Design review of the part built by this model. Coordinates are the model's own, in mm. Round coordinates to 2 decimals unless told otherwise and drop trailing zeros. Return JSON: item names as keys, results as strings. Group by question number.
(1) Clearance check with a flat-ended pin moving along its axis: pin 1 (6 mm diameter, centred on x = 87.5, z = 87.5, fed in from +Y). State where the tip first meets the part, or that it passes through.
(2) Wall thickness on L1, parallel to X at y = 0.55, z = -87.5: over which ranges is the line inside the solid? List them lowest first. Write a range as [from, to].
(3) The part is to be moulded in two halves that separate along Z. For faces 1 (the conical face through (-90.063, 1.125, -88.069)), 2 (the conical face through (-90.063, 1.125, 86.931)), 3 (the cylindrical face through (116, 1.48, -116.07)), 4 (the flat face through (2, 0, -2)), say which applies: pulls with the +Z half, pulls with the -Z half, needs draft (parallel to the pull), parting line crosses it, or undercut.
from build123d import *

# Parameters (mm, degrees)
ESQUISSE1_R        = 2.5
BOSS_EXTRU_1_DEPTH = 3
CHANFREIN1_SIZE    = 2


with BuildPart() as part:
    # Esquisse1 → Boss.-Extru.1 (new body)
    with BuildSketch(Plane(origin=(0, 0, 0), x_dir=(1, 0, 0), z_dir=(0, 1, 0))):
        with BuildLine():
            Line((112.5, -117.5), (-112.5, -117.5))
            ThreePointArc((-112.5, -117.5), (-116.035533906, -116.035533906), (-117.5, -112.5))
            Line((-117.5, -112.5), (-117.5, 112.5))
            ThreePointArc((-117.5, 112.5), (-116.035533906, 116.035533906), (-112.5, 117.5))
            Line((-112.5, 117.5), (112.5, 117.5))
            ThreePointArc((112.5, 117.5), (116.035533906, 116.035533906), (117.5, 112.5))
            Line((117.5, 112.5), (117.5, -112.5))
            ThreePointArc((117.5, -112.5), (116.035533906, -116.035533906), (112.5, -117.5))
        make_face()
        with Locations(Location((-87.5, 87.5, 0), (0, 0, 270))):
            Circle(ESQUISSE1_R, mode=Mode.SUBTRACT)
        with Locations(Location((-87.5, -87.5, 0), (0, 0, 270))):
            Circle(ESQUISSE1_R, mode=Mode.SUBTRACT)
        with Locations(Location((87.5, -87.5, 0), (0, 0, 270))):
            Circle(ESQUISSE1_R, mode=Mode.SUBTRACT)
        with Locations(Location((87.5, 87.5, 0), (0, 0, 270))):
            Circle(ESQUISSE1_R, mode=Mode.SUBTRACT)
    extrude(amount=BOSS_EXTRU_1_DEPTH)

    # Chanfrein1
    chanfrein1_edges = [part.edges().sort_by_distance(p)[0] for p in [
        (-87.5, 3, -90),
        (-87.5, 3, 85),
        (87.5, 3, 85),
        (87.5, 3, -90),
    ]]
    chamfer(chanfrein1_edges, length=CHANFREIN1_SIZE)


solid = part.part
Solutions:
{
 "1": {"pin 1": "y = 1.5"},
 "2": {"L1": "[-117.5, -90], [-85, 85], [90, 117.5]"},
 "3": {"face 1": "undercut", "face 2": "undercut", "face 3": "pulls with the -Z half", "face 4": "needs draft"}
}
